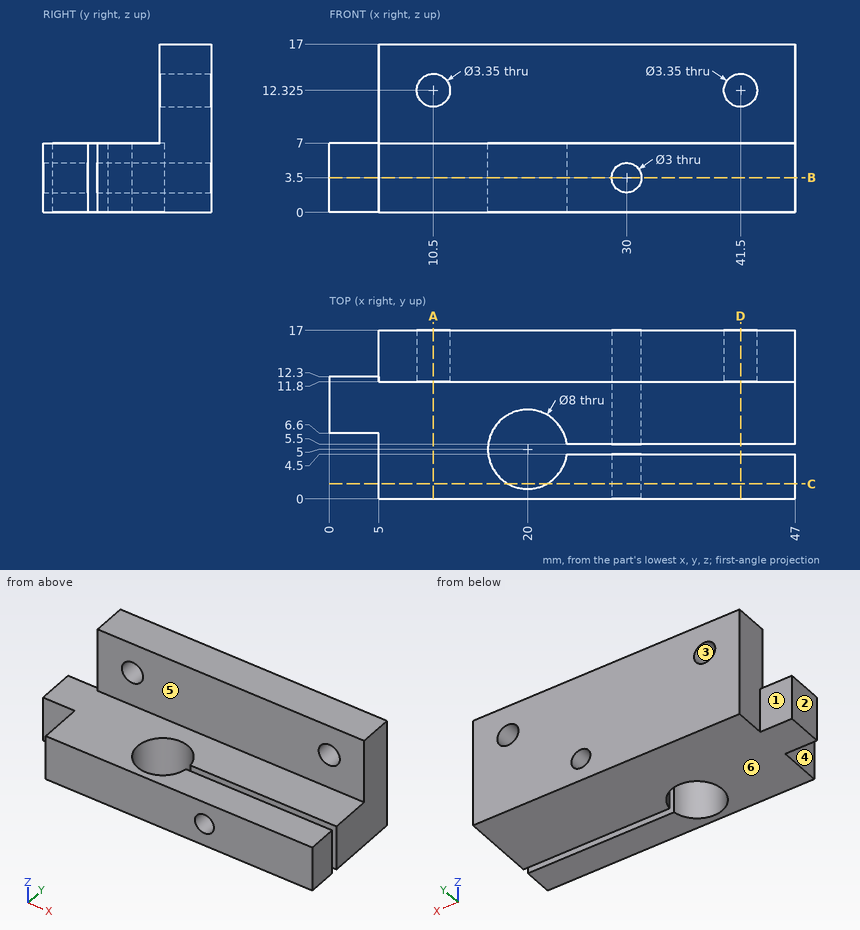
The drawing under review shows one solid part. Ordinate dimensions are in mm from its lowest x, y, z. A direction names the side the tool comes from. Give positions to 0.01 mm unless a question says otherwise; leave off trailing zeros. Loops run counter-clockwise (first coordinate to the right, second up) from the corner with the lowest first, then second, coordinate; pieces in that order, holes last. Notation, with made-up numbers: M 37,27.25 L 53,27.25 A13 cw 53,40.25 Z; hole C 76,88 d9. An arc over 180 degrees is marked long. Return JSON: item names as keys, results as strings. Group by question number.
Item 1: We need section D-D (x = 41.5). Give the boundary of the cut face in (y, z), and give its area (3 significant figures).
Item 2: Tool access review of the marked faces 4, 5 and 6: name each direction out of +Z, -Z, +X, -X, +Y, -Y from which nothing blocks a thin tool from reaching the whole face with its end or side.
Item 3: Mouldability with a two-part tool opening along X and no side actions: class the marked faces 1, 2 and 3 as released by +X, released by -X, zero draft, split by the parting line, or undercut.
Item 4: We need section B-B (z = 3.5). Give the boundary of the cut face in (x, y), and give its area (3 significant figures).
Item 5: Insertion check: pin 1 Ø4 at (x, z) = (1.5, 2.5) entering from +Y; pin 2 Ø5.5 at (x, z) = (2, 2.5) entering from -Y; pin 3 Ø4 at (x, z) = (25.5, 13) entering from -Y; pin 4 Ø5 at (x, y) = (39.5, 10.5) entering from +Z. Each pin has a flat end and moves straight along its axis. Give the tip position at first contact, or say it passes through.
Item 6: We need section A-A (x = 10.5). Give the boundary of the cut face in (y, z).
Item 7: For probe 1 along Z at (x, y) = (30, 0.9); probe 2 along X at (y, z) = (2.5, 4.25); probe 3 along Y at (x, z) = (45, 1.25), list the stretches that pass through material, from the lowest coordinate up.
Item 8: We need section C-C (y = 1.5). Give the boundary of the cut face in (x, z).
Output:
{
 "1": {"outline": "M 0,0 L 4.5,0 L 4.5,7 L 0,7 Z; M 5.5,0 L 17,0 L 17,10.65 L 11.8,10.65 L 11.8,7 L 5.5,7 Z; M 11.8,14 L 17,14 L 17,17 L 11.8,17 Z", "area": "147 mm^2"},
 "2": {"face 4": "+Z, -Z, -X, -Y", "face 5": "+Z, +X, -X, -Y", "face 6": "-Z, +X, -X, +Y, -Y"},
 "3": {"face 1": "zero draft", "face 2": "released by -X", "face 3": "undercut"},
 "4": {"outline": "M 0,6.6 L 5,6.6 L 5,0 L 28.5,0 L 28.5,4.5 L 23.97,4.5 A4 cw long 23.97,5.5 L 28.5,5.5 L 28.5,17 L 5,17 L 5,12.3 L 0,12.3 Z; M 31.5,0 L 47,0 L 47,4.5 L 31.5,4.5 Z; M 31.5,5.5 L 47,5.5 L 47,17 L 31.5,17 Z", "area": "621 mm^2"},
 "5": {"pin 1": "stops at y = 12.3", "pin 2": "stops at y = 6.6", "pin 3": "stops at y = 11.8", "pin 4": "stops at z = 17"},
 "6": {"outline": "M 0,0 L 17,0 L 17,10.65 L 11.8,10.65 L 11.8,7 L 0,7 Z; M 11.8,14 L 17,14 L 17,17 L 11.8,17 Z"},
 "7": {"probe 1": "z = 0 to 2, 5 to 7", "probe 2": "x = 5 to 16.88, 23.12 to 28.7, 31.3 to 47", "probe 3": "y = 0 to 4.5, 5.5 to 17"},
 "8": {"outline": "M 5,0 L 18.06,0 L 18.06,7 L 5,7 Z; M 21.94,0 L 47,0 L 47,7 L 21.94,7 Z; hole C 30,3.5 d3"}
}
